The listing builds one solid part. Answer for the finished solid, in the listing's coordinates (mm). Face numbers are marked on the shaded views. A direction names the side the tool comes from. Coordinates: 2 decimals unless noted, no trailing zeros. Write each loop counter-clockwise with the first axis right and the second up, starting at its lowest first coordinate (ties: lowest second). Pieces come first, ordered by that corner, then holes.
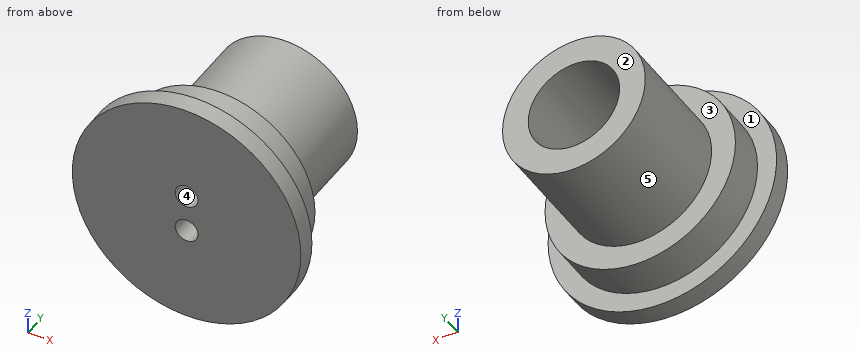
from build123d import *

# Parameters (mm, degrees)
SKETCH1_R               = 6.35
BOSS_EXTRUDE1_DEPTH     = 2.54
SKETCH2_R               = 4.7625
BOSS_EXTRUDE2_DEPTH     = 7.62
SKETCH3_R               = 3.048
CUT_EXTRUDE1_DEPTH      = 7.62
SKETCH6_R               = 7.62
BOSS_EXTRUDE3_DEPTH     = 1.27
SKETCH4_R               = 0.762
CUT_EXTRUDE2_DEPTH      = 8.62
CUT_EXTRUDE2_DEPTH_BACK = 4.81
SKETCH5_R               = 0.762
CUT_EXTRUDE3_DEPTH      = 4.81


with BuildPart() as part:
    # Sketch1 → Boss-Extrude1 (new body)
    with BuildSketch(Plane(origin=(0, 0, 0), x_dir=(1, 0, 0), z_dir=(0, 1, 0))):
        Circle(SKETCH1_R)
    extrude(amount=BOSS_EXTRUDE1_DEPTH)

    # Sketch2 → Boss-Extrude2 (add)
    with BuildSketch(Plane(origin=(0, 2.54, 0), x_dir=(1, 0, 0), z_dir=(0, 1, 0))):
        Circle(SKETCH2_R)
    extrude(amount=BOSS_EXTRUDE2_DEPTH)

    # Sketch3 → Cut-Extrude1 (cut)
    with BuildSketch(Plane(origin=(0, 10.16, 0), x_dir=(1, 0, 0), z_dir=(0, 1, 0))):
        Circle(SKETCH3_R)
    extrude(amount=-CUT_EXTRUDE1_DEPTH, mode=Mode.SUBTRACT)

    # Sketch6 → Boss-Extrude3 (add)
    with BuildSketch(Plane.XZ):
        Circle(SKETCH6_R)
    extrude(amount=BOSS_EXTRUDE3_DEPTH)

    # Sketch4 → Cut-Extrude2 (cut, two sides)
    with BuildSketch(Plane(origin=(0, 2.54, 0), x_dir=(1, 0, 0), z_dir=(0, 1, 0))) as cut_extrude2_sk:
        with Locations((0, -1.27)):
            Circle(SKETCH4_R)
    extrude(amount=CUT_EXTRUDE2_DEPTH, mode=Mode.SUBTRACT)
    extrude(cut_extrude2_sk.sketch, amount=-CUT_EXTRUDE2_DEPTH_BACK, mode=Mode.SUBTRACT)

    # Sketch5 → Cut-Extrude3 (cut, through all)
    with BuildSketch(Plane(origin=(0, 2.54, 0), x_dir=(1, 0, 0), z_dir=(0, 1, 0))):
        with Locations((0, 1.27)):
            Circle(SKETCH5_R)
    extrude(amount=-CUT_EXTRUDE3_DEPTH, mode=Mode.SUBTRACT)


solid = part.part
1. Section A-A on x = 0 is taken. Give the vertices of the cut face in (y, z).
Results found:
outline: (-1.27, -7.62) - (0, -7.62) - (0, -6.35) - (2.54, -6.35) - (2.54, -4.76) - (10.16, -4.76) - (10.16, -3.05) - (2.54, -3.05) - (2.54, -2.03) - (-1.27, -2.03) - close; (-1.27, -0.51) - (2.54, -0.51) - (2.54, 0.51) - (-1.27, 0.51) - close; (-1.27, 2.03) - (2.54, 2.03) - (2.54, 3.05) - (10.16, 3.05) - (10.16, 4.76) - (2.54, 4.76) - (2.54, 6.35) - (0, 6.35) - (0, 7.62) - (-1.27, 7.62) - close
2. Section C-C on y = 1.5 is taken. Give the vertices of the cut face in (x, z), then the cut area to 3 significant figures.
Results found:
outline: circle Ø12.7 at (0, 0); hole circle Ø1.52 at (0, -1.27); hole circle Ø1.52 at (0, 1.27)
area: 123 mm2
3. Find the intervals of material crossed by L1, parallel to Z at x = 0, y = 0.5; L2, parallel to Z at x = 0, y = 6, in increasing order.
Results found:
L1: z = -6.35 to -2.03, -0.51 to 0.51, 2.03 to 6.35
L2: z = -4.76 to -3.05, 3.05 to 4.76
4. Section D-D on z = -5 is taken. Give the vertices of the cut face in (x, y), then the cut area to 3 significant figures.
Results found:
outline: (-5.75, -1.27) - (5.75, -1.27) - (5.75, 0) - (3.91, 0) - (3.91, 2.54) - (-3.91, 2.54) - (-3.91, 0) - (-5.75, 0) - close
area: 34.5 mm2
5. Section B-B on z = 1.27 is taken. Give the vertices of the cut face in (x, y), then the cut area to 3 significant figures.
Results found:
outline: (-7.51, -1.27) - (-0.76, -1.27) - (-0.76, 2.54) - (-2.77, 2.54) - (-2.77, 10.16) - (-4.59, 10.16) - (-4.59, 2.54) - (-6.22, 2.54) - (-6.22, 0) - (-7.51, 0) - close; (0.76, -1.27) - (7.51, -1.27) - (7.51, 0) - (6.22, 0) - (6.22, 2.54) - (4.59, 2.54) - (4.59, 10.16) - (2.77, 10.16) - (2.77, 2.54) - (0.76, 2.54) - close
area: 72.6 mm2
6. For a pull along X with two mould halves and no side action, classify the marked faces 3, 4 and 5 as pulls with the +X half, pulls with the -X half, needs draft (parallel to the pull), parting line crosses it, or undercut.
Results found:
face 3: needs draft
face 4: undercut
face 5: parting line crosses it
7. Flat-ended cylindrical pins translate along their axes: P1, Ø1, axis at x = -4.5, y = 4.5, coming from the +Z side; P2, Ø2.5, axis at x = 0, z = 1.27, coming from the +Y side; P3, Ø3, axis at y = 7, z = 4.5, coming from the +X side. Find the tip coordinate at first contact, or state that the pin passes through.
Results found:
P1: stops at z = 2.58
P2: stops at y = 2.54
P3: stops at x = 3.7
8. A tool of negligible diameter and unlimited length cuts with its end or side. For the marked faces 1 and 2, from which of +Z, -Z, +X, -X, +Y, -Y can it reach the whole face along a straight path? Write none if from no direction.
Results found:
face 1: +Y
face 2: +Z, -Z, +X, -X, +Y
